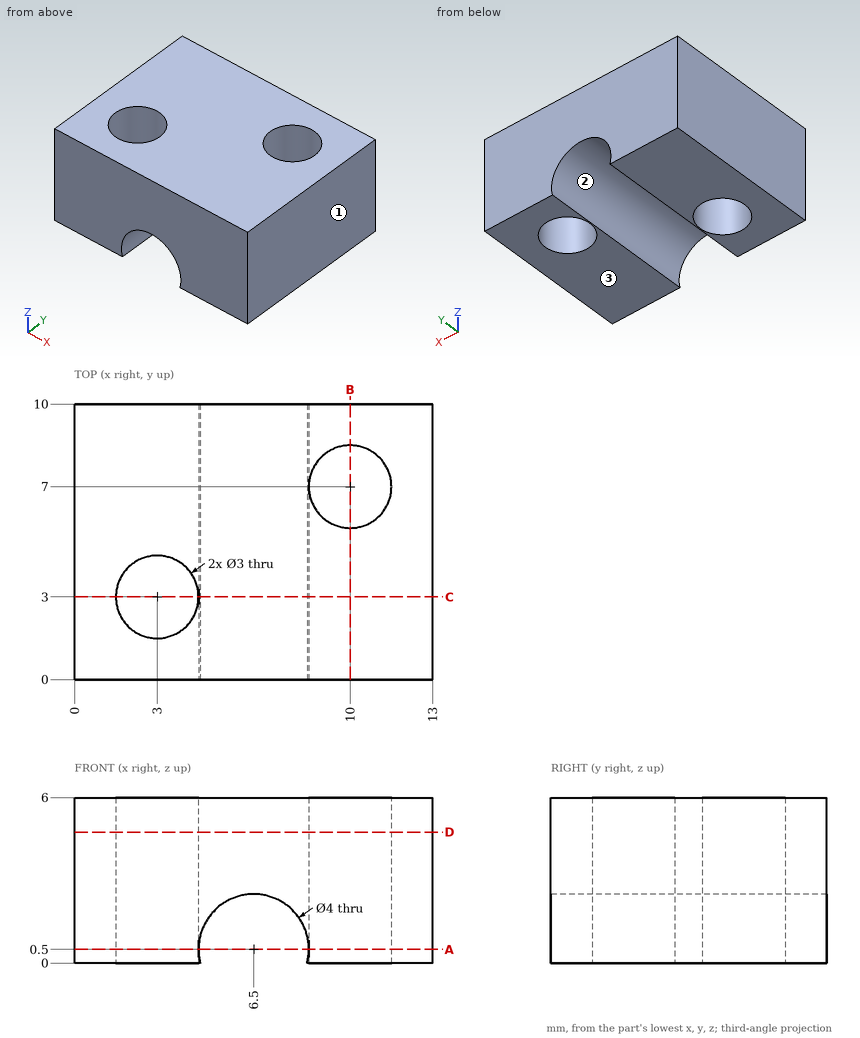
Check sheet for the drawn part. Datum: minimum x, y, z corner. Units: mm. Round coordinates to 2 decimals unless told otherwise and drop trailing zeros. Loops run counter-clockwise (first coordinate to the right, second up) from the corner with the lowest first, then second, coordinate; pieces in that order, holes last. Notation, with made-up numbers: (46, -35) -> (93, -35) arc R5 cw to (93, -30) -> close; hole circle Ø1 at (-4.75, 44). An arc over 180 degrees is marked (long way). Put each result on its own line as item: value. Start each with the question number.
1. Section check C-C (y = 3). Enter the section's corners in (x, z).
2. Gauge pin test, flat end, axial feed: pin 1 (2.5 mm diameter, centred on x = 6.5, z = 0.5, fed in from +Y). Record the tip position at first contact, or that the pin passes through.
3. Draft check along Z on the marked faces 1, 2 and 3. Enter one of: +Z half, -Z half, draft (parallel to the pull), parting line (faces both ways), or undercut.
4. Section check B-B (x = 10). Enter the section's corners in (y, z), plus the area to 3 significant figures.
5. Section check A-A (z = 0.5). Enter the section's corners in (x, y), plus the area to 3 significant figures.
6. Section check D-D (z = 4.75). Enter the section's corners in (x, y), plus the area to 3 significant figures.
7. Scan lines: probe 1 along Y at (x, z) = (10, 4.2); probe 2 along X at (y, z) = (2.5, 2.1); probe 3 along X at (y, z) = (4, 1.8). Record each from-to range of solid material in increasing order.
Findings:
1. outline: (0, 0) -> (1.5, 0) -> (1.5, 6) -> (0, 6) -> close; (4.5, 0) -> (4.56, 0) arc R2 cw (long way) to (8.44, 0) -> (13, 0) -> (13, 6) -> (4.5, 6) -> close
2. pin 1: passes through
3. face 1: draft
3. face 2: undercut
3. face 3: -Z half
4. outline: (0, 0) -> (5.5, 0) -> (5.5, 6) -> (0, 6) -> close; (8.5, 0) -> (10, 0) -> (10, 6) -> (8.5, 6) -> close
4. area: 42.0 mm^2
5. outline: (0, 0) -> (4.5, 0) -> (4.5, 10) -> (0, 10) -> close; (8.5, 0) -> (13, 0) -> (13, 10) -> (8.5, 10) -> close; hole circle Ø3 at (3, 3); hole circle Ø3 at (10, 7)
5. area: 75.9 mm^2
6. outline: (0, 0) -> (13, 0) -> (13, 10) -> (0, 10) -> close; hole circle Ø3 at (3, 3); hole circle Ø3 at (10, 7)
6. area: 116 mm^2
7. probe 1: y = 0 to 5.5, 8.5 to 10
7. probe 2: x = 0 to 1.59, 4.41 to 5.3, 7.7 to 13
7. probe 3: x = 0 to 1.88, 4.12 to 4.98, 8.02 to 13
